from build123d import *

# Parameters (mm, degrees)
SKETCH1_R           = 17
SKETCH1_R_2         = 1.55
SKETCH1_R_3         = 1.05
SKETCH1_R_4         = 8
BOSS_EXTRUDE1_DEPTH = 7
SKETCH2_R           = 3
CUT_EXTRUDE2_DEPTH  = 2.5


with BuildPart() as part:
    # Sketch1 → Boss-Extrude1 (new body)
    with BuildSketch(Plane.XY):
        Circle(SKETCH1_R)
        with Locations((0, 12.5)):
            Circle(SKETCH1_R_2, mode=Mode.SUBTRACT)
        with Locations((12.5, 0)):
            Circle(SKETCH1_R_2, mode=Mode.SUBTRACT)
        with Locations((0, -12.5)):
            Circle(SKETCH1_R_2, mode=Mode.SUBTRACT)
        with Locations((-12.5, 0)):
            Circle(SKETCH1_R_2, mode=Mode.SUBTRACT)
        with Locations((-8.980256121, 8.980256121)):
            Circle(SKETCH1_R_3, mode=Mode.SUBTRACT)
        with Locations((8.980256121, 8.980256121)):
            Circle(SKETCH1_R_3, mode=Mode.SUBTRACT)
        with Locations((8.980256121, -8.980256121)):
            Circle(SKETCH1_R_3, mode=Mode.SUBTRACT)
        with Locations((-8.980256121, -8.980256121)):
            Circle(SKETCH1_R_3, mode=Mode.SUBTRACT)
        Circle(SKETCH1_R_4, mode=Mode.SUBTRACT)
    extrude(amount=BOSS_EXTRUDE1_DEPTH)

    # Sketch2 → Cut-Extrude2 (cut)
    with BuildSketch(Plane.XY.offset(7)):
        with Locations((0, 12.5)):
            Circle(SKETCH2_R)
        with Locations((12.5, 0)):
            Circle(SKETCH2_R)
        with Locations((0, -12.5)):
            Circle(SKETCH2_R)
        with Locations((-12.5, 0)):
            Circle(SKETCH2_R)
    extrude(amount=-CUT_EXTRUDE2_DEPTH, mode=Mode.SUBTRACT)


solid = part.part
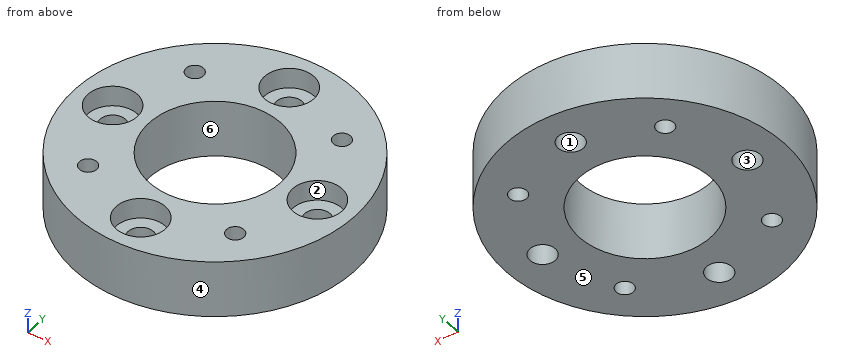
Source: CAD feature listing. Evaluate the final solid. Frame: model axes, mm. Face numbers are marked on the shaded views. A direction names the side the tool comes from. Round coordinates to 2 decimals unless told otherwise and drop trailing zeros. Order: outer loops, then holes, each group sorted by start corner. A loop starts at its lowest first (then second) coordinate and runs counter-clockwise, first axis right, second up. Notation, with made-up numbers: (49, 52) - (108, 52) arc R24 cw to (108, 75) - close; hole circle Ø11 at (64, -4.75). An arc over 180 degrees is marked (long way). Use a Markdown table: item, result. Add a question column.
1. First-contact query: pin 1 (4 mm diameter, centred on y = 5.5, z = 5.5, fed in from -X); pin 2 (4 mm diameter, centred on y = -6, z = 4, fed in from -X); pin 3 (1.8 mm diameter, centred on x = -0.5, y = -11.5, fed in from +Z). Flat tips, straight axial feed; report the tip coordinate or a pass-through.
2. Line query: probe 1 along Y at (x, z) = (0, 3.55); probe 2 along X at (y, z) = (1, 4); probe 3 along Y at (x, z) = (0, 6). Output: solid intervals per line, ascending.
3. Section query C-C (z = 5.5). Give the number of separate pieces and of enclosed holes in the cut face, then the cut area to 3 significant figures.
4. Section query A-A (y = 0). Return the cut outline in (x, z).
5. Section query D-D (x = 2). Return the cut outline in (y, z).
6. Section query B-B (y = 11.5). Return the cut outline in (x, z), then the cut area to 3 significant figures.
7. Set-up query: the marked faces 1 and 2. Return all of +Z, -Z, +X, -X, +Y, -Y with unobstructed straight access to the full face (end or side cutting, diameter ignored); none if empty.
8. Mould query, pull axis Y, two halves, no side actions, for the marked faces 3, 4, 5 and 6. Classes: +Y half, -Y half, draft (parallel to the pull), parting line (faces both ways), or undercut.
Derived:
| question | item | result |
|---|---|---|
| 1 | pin 1 | x = -16.64 |
| 1 | pin 2 | x = -16.52 |
| 1 | pin 3 | z = 4.5 |
| 2 | probe 1 | -17 to -14.05, -10.95 to -8, 8 to 10.95, 14.05 to 17 |
| 2 | probe 2 | -16.97 to -13.68, -11.32 to -7.94, 7.94 to 11.32, 13.68 to 16.97 |
| 2 | probe 3 | -17 to -15.5, -9.5 to -8, 8 to 9.5, 15.5 to 17 |
| 3 | separate pieces | 1 |
| 3 | enclosed holes | 9 |
| 3 | area | 580 mm2 |
| 4 | outline | (-17, 0) - (-14.05, 0) - (-14.05, 4.5) - (-15.5, 4.5) - (-15.5, 7) - (-17, 7) - close; (-10.95, 0) - (-8, 0) - (-8, 7) - (-9.5, 7) - (-9.5, 4.5) - (-10.95, 4.5) - close; (8, 0) - (10.95, 0) - (10.95, 4.5) - (9.5, 4.5) - (9.5, 7) - (8, 7) - close; (14.05, 0) - (17, 0) - (17, 7) - (15.5, 7) - (15.5, 4.5) - (14.05, 4.5) - close |
| 5 | outline | (-16.88, 0) - (-7.75, 0) - (-7.75, 7) - (-10.26, 7) - (-10.26, 4.5) - (-14.74, 4.5) - (-14.74, 7) - (-16.88, 7) - close; (7.75, 0) - (16.88, 0) - (16.88, 7) - (14.74, 7) - (14.74, 4.5) - (10.26, 4.5) - (10.26, 7) - (7.75, 7) - close |
| 6 | outline | (-12.52, 0) - (-1.18, 0) - (-1.18, 4.5) - (-2.83, 4.5) - (-2.83, 7) - (-12.52, 7) - close; (1.18, 0) - (12.52, 0) - (12.52, 7) - (2.83, 7) - (2.83, 4.5) - (1.18, 4.5) - close |
| 6 | area | 150 mm2 |
| 7 | face 1 | +Z, -Z |
| 7 | face 2 | +Z |
| 8 | face 3 | undercut |
| 8 | face 4 | parting line |
| 8 | face 5 | draft |
| 8 | face 6 | undercut |
